from build123d import *

# Parameters (mm, degrees)
BOSS_EXTRUDE1_DEPTH = 3
SKETCH3_W           = 5.2
SKETCH3_H           = 3.2
SKETCH3_W_2         = 10.2
SKETCH3_W_3         = 30.2
SKETCH3_W_4         = 3.2
SKETCH3_H_2         = 10.2
CUT_EXTRUDE1_DEPTH  = 4


with BuildPart() as part:
    # Sketch1 → Boss-Extrude1 (new body)
    with BuildSketch(Plane(origin=(0, 0, 0), x_dir=(1, 0, 0), z_dir=(0, 1, 0))):
        Polygon((0, 0), (75, 0), (75, -15), (15, -15), (15, -139.694434203), (0, -139.694434203), align=None)
    extrude(amount=-BOSS_EXTRUDE1_DEPTH)

    # Sketch3 → Cut-Extrude1 (cut, through all)
    with BuildSketch(Plane(origin=(0, 0, 0), x_dir=(1, 0, 0), z_dir=(0, 1, 0))):
        with Locations((2.5, -138.194434203)):
            Rectangle(SKETCH3_W, SKETCH3_H)
        with Locations((15, -1.5)):
            Rectangle(SKETCH3_W_2, SKETCH3_H)
        with Locations((45, -1.5)):
            Rectangle(SKETCH3_W_3, SKETCH3_H)
        with Locations((13.5, -104.694434203)):
            Rectangle(SKETCH3_W_4, SKETCH3_H_2)
        with Locations((13.5, -64.694434203)):
            Rectangle(SKETCH3_W_4, SKETCH3_H_2)
        with Locations((13.5, -124.694434203)):
            Rectangle(SKETCH3_W_4, SKETCH3_H_2)
        with Locations((13.5, -44.694434203)):
            Rectangle(SKETCH3_W_4, SKETCH3_H_2)
        with Locations((13.5, -24.694434203)):
            Rectangle(SKETCH3_W_4, SKETCH3_H_2)
        with Locations((13.5, -84.694434203)):
            Rectangle(SKETCH3_W_4, SKETCH3_H_2)
        Polygon((75.1, 0.1), (64.9, 0.1), (64.9, -3.1), (71.15, -3.1), (71.15, -10.1), (74.4, -10.1), (74.4, -15.1), (75.1, -15.1), align=None)
    extrude(amount=-CUT_EXTRUDE1_DEPTH, mode=Mode.SUBTRACT)


solid = part.part
Geometry check sheet. Reference: the model listing, model coordinates, mm. A direction names the side the tool comes from. Give positions to 0.01 mm unless a question says otherwise; leave off trailing zeros. Loops run counter-clockwise (first coordinate to the right, second up) from the corner with the lowest first, then second, coordinate; pieces in that order, holes last.
(1) Set-up check for faces 1 (the flat face through (60.1, -1, 2)), 2 (the flat face through (13, -1, 89.794)), 3 (the flat face through (15, -1, 55)): record each of +Z, -Z, +X, -X, +Y, -Y from which the full face is reachable in a straight line by a thin tool's end or side.
From the geometry:
face 1: -Z, +Y, -Y
face 2: +X, +Y, -Y
face 3: +Z, +X, +Y, -Y
(2) Section check A-A on z = 61. Record the cut outline in (x, y).
From the geometry:
outline: (0, -3) - (11.9, -3) - (11.9, 0) - (0, 0) - close
(3) Thickness scan on L1, parallel to X at y = -1.7, z = 68.5; L2, parallel to X at y = -0.5, z = 78; L3, parallel to Z at x = 42, y = -2.8. Record the ranges inside material, lowest first.
From the geometry:
L1: x = 0 to 11.9
L2: x = 0 to 15
L3: z = 3.1 to 15
(4) Section check B-B on x = 53. Record the cut outline in (y, z).
From the geometry:
outline: (-3, 3.1) - (0, 3.1) - (0, 15) - (-3, 15) - close
(5) Depth check by flat-ended pin: pin 1 Ø1.5 at (y, z) = (-2, 95) entering from +X; pin 2 Ø1.5 at (x, y) = (14, -1) entering from -Z; pin 3 Ø0.9 at (x, y) = (73, -1.5) entering from -Z; pin 4 Ø1 at (y, z) = (-1, 42.5) entering from -X. Enter the tip coordinate at first touch or a pass-through.
From the geometry:
pin 1: stops at x = 15
pin 2: stops at z = 3.1
pin 3: stops at z = 10.1
pin 4: stops at x = 0
